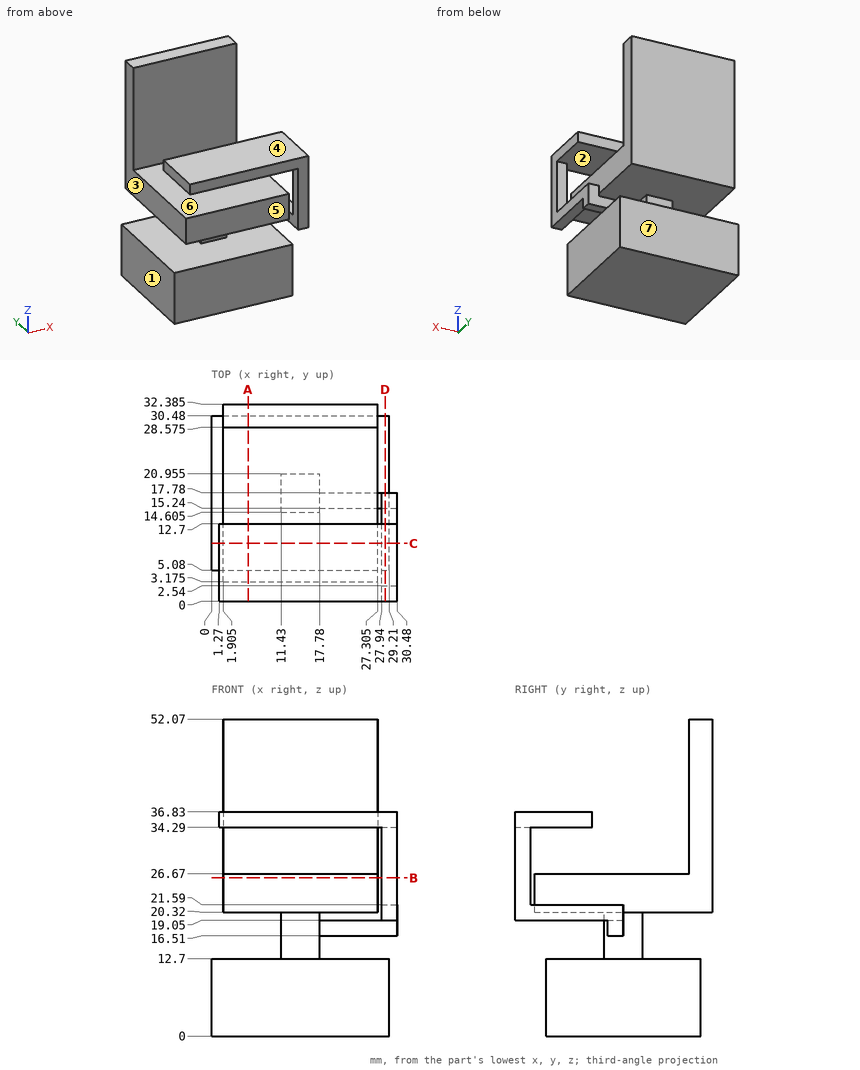
Source: three-view drawing plus pictorial views. Frame: mm from the lowest corner of the part. A direction names the side the tool comes from. Round coordinates to 2 decimals unless told otherwise and drop trailing zeros. Loops run counter-clockwise (first coordinate to the right, second up) from the corner with the lowest first, then second, coordinate; pieces in that order, holes last. Notation, with made-up numbers: M 54.25,-7.5 L 97.25,-7.5 A9 ccw 97.25,1.5 Z; hole C 62,-12.75 d10. An arc over 180 degrees is marked long. Put each result on its own line as item: value. Start each with the question number.
(1) Draft query along Z for the marked faces 1, 2, 3 and 4. Return one class per face: +Z half, -Z half, draft (parallel to the pull), parting line (faces both ways), or undercut.
(2) Section query B-B (z = 26). Return loops of the section in (x, y) (3 decimals), then the cut area to 3 significant figures.
(3) Set-up query: the marked faces 5, 6 and 7. Return all of +Z, -Z, +X, -X, +Y, -Y with unobstructed straight access to the full face (end or side cutting, diameter ignored); none if empty.
(4) Section query D-D (x = 28.5). Return loops of the section in (y, z), then the cut area to 3 significant figures.
(5) Contact query for flat-ended pins moving along their axis: pin 1 Ø12.5 at (x, y) = (8.5, 15) entering from +Z; pin 2 Ø5 at (x, z) = (13.5, 15.5) entering from -Y (3 decimals); pin 3 Ø10 at (y, z) = (23.5, 7.5) entering from +X. Output: stop coordinate, or through.
(6) Section query C-C (y = 9.5). Return loops of the section in (x, z) (3 decimals).
(7) Material intervals for line 1 along Z through (x, y) = (10, 12.5); line 2 along Z through (x, y) = (5.5, 18.5); line 3 along Z through (x, y) = (3, 4), sorted ascending. Write a range as [from, to].
(8) Section query A-A (x = 6). Return loops of the section in (y, z) (3 decimals).
Findings below:
1. face 1: draft
1. face 2: undercut
1. face 3: undercut
1. face 4: +Z half
2. outline: M 1.905,3.175 L 27.305,3.175 L 27.305,32.385 L 1.905,32.385 Z; M 27.94,0 L 30.48,0 L 30.48,2.54 L 27.94,2.54 Z
2. area: 748 mm2
3. face 5: -Z, -X, -Y
3. face 6: +X, -X, -Y
3. face 7: -Z, +X, -X, +Y
4. outline: M 0,19.05 L 15.24,19.05 L 15.24,16.51 L 17.78,16.51 L 17.78,21.59 L 2.54,21.59 L 2.54,34.29 L 12.7,34.29 L 12.7,36.83 L 0,36.83 Z; M 5.08,0 L 30.48,0 L 30.48,12.7 L 5.08,12.7 Z
4. area: 439 mm2
5. pin 1: stops at z = 36.83
5. pin 2: stops at y = 14.605
5. pin 3: stops at x = 29.21
6. outline: M 0,0 L 29.21,0 L 29.21,12.7 L 0,12.7 Z; M 1.27,34.29 L 30.48,34.29 L 30.48,36.83 L 1.27,36.83 Z; M 1.905,20.32 L 27.305,20.32 L 27.305,26.67 L 1.905,26.67 Z; M 27.94,19.05 L 30.48,19.05 L 30.48,21.59 L 27.94,21.59 Z
7. line 1: z = [0, 12.7], [20.32, 26.67], [34.29, 36.83]
7. line 2: z = [0, 12.7], [20.32, 26.67]
7. line 3: z = [20.32, 26.67], [34.29, 36.83]
8. outline: M 0,34.29 L 12.7,34.29 L 12.7,36.83 L 0,36.83 Z; M 3.175,20.32 L 32.385,20.32 L 32.385,52.07 L 28.575,52.07 L 28.575,26.67 L 3.175,26.67 Z; M 5.08,0 L 30.48,0 L 30.48,12.7 L 5.08,12.7 Z
